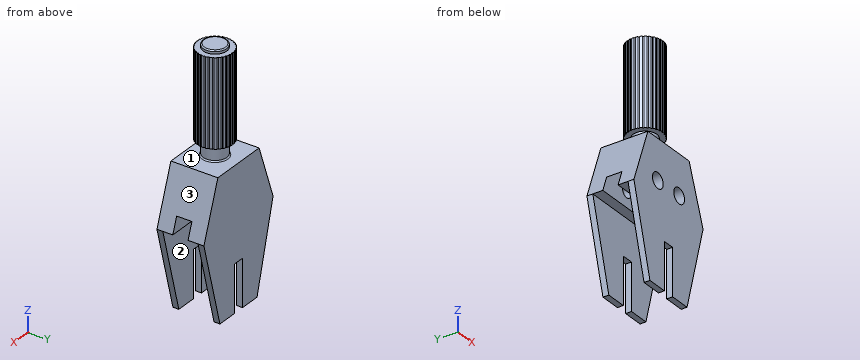
```python
from build123d import *

# Parameters (mm, degrees)
F1_DEPTH         = 200
F2_R             = 100
F3_DEPTH         = 900
F5_R             = 150
F6_DEPTH         = 740
F8_DEPTH         = 580
F9_R             = 65
F9_R_2           = 50
F10_DEPTH        = 100
F11_DEPTH        = 350
F13_DEPTH        = 65
F14_R            = 10
F15_W            = 11.6287115961
F15_H            = 9.4758689404
F16_DEPTH        = 740
F16_COPIES_COUNT = 30


# Not quite as in the source:
# - a pattern or mirror of a feature is missing from the dataset's text; its kind, count and spacing are read off the source's solid


with BuildPart() as f1:
    # F0 (on Front) → F1 (new body, symmetric)
    with BuildSketch(Plane.XZ):
        Polygon((250, 794.9763654469), (-250, 794.9763654469), (-419.1142838269, 324.4443697168), (-225, -400), (-50, -400), (-50, 0), (0, 0), (50, 0), (50, -400), (225, -400), (419.1142838269, 324.4443697168), align=None)
    extrude(amount=F1_DEPTH, both=True)

    # F2 (on face) → F3 (join)
    with BuildSketch(Plane.XY.offset(794.9763654469)):
        Circle(F2_R)
    extrude(amount=F3_DEPTH)

    # F5 (on offset) → F6 (join)
    with BuildSketch(Plane.XY.offset(924.9763654469)):
        Circle(F5_R)
    extrude(amount=F6_DEPTH)

    # F7 (on Right) → F8 (cut, symmetric)
    with BuildSketch(Plane.YZ):
        Polygon((-150, 324.4443697168), (-150, -400), (150, -400), (150, 324.4443697168), (65, 324.4443697168), (65, 454.4443697168), (-65, 454.4443697168), (-65, 324.4443697168), align=None)
    extrude(amount=F8_DEPTH, both=True, mode=Mode.SUBTRACT)

    # F9 (on face) → F10 (cut)
    with BuildSketch(Plane.XZ.offset(200)):
        with Locations((-129.1142838269, 454.4443697168)):
            Circle(F9_R)
        with Locations((-129.1142838269, 454.4443697168)):
            Circle(F9_R_2, mode=Mode.SUBTRACT)
        with Locations((129.1142838269, 454.4443697168)):
            Circle(F9_R)
        with Locations((129.1142838269, 454.4443697168)):
            Circle(F9_R_2, mode=Mode.SUBTRACT)
    extrude(amount=-F10_DEPTH, mode=Mode.SUBTRACT)

    # F11 (cut): faces of the model
    f11_faces = [f1.faces().sort_by_distance(p)[0] for p in [
        (-129.1142838269, -200, 454.4443697168),
        (129.1142838269, -200, 454.4443697168),
    ]]
    extrude(f11_faces, amount=-F11_DEPTH, mode=Mode.SUBTRACT)

    # F12 (on Front) → F13 (cut, symmetric)
    with BuildSketch(Plane.XZ):
        Polygon((272.5361245925, 584.4443697168), (-272.5361245925, 584.4443697168), (-297.6948810114, 514.4443697168), (-372.3908790489, 454.4443697168), (-419.1142838269, 324.4443697168), (419.1142838269, 324.4443697168), (372.3908790489, 454.4443697168), (297.6948810114, 514.4443697168), align=None)
    extrude(amount=F13_DEPTH, both=True, mode=Mode.SUBTRACT)

    # F14
    f14_edges = [f1.edges().sort_by_distance(p)[0] for p in [
        (-100, 0, 1694.976365),
        (-100, 0, 794.976365),
    ]]
    fillet(f14_edges, radius=F14_R)

    # F15 (on face) → F16 (cut, through all)
    with BuildSketch(Plane.XY.offset(1664.9763654469)):
        with Locations((0, 150)):
            Rectangle(F15_W, F15_H)
    f16 = extrude(amount=-F16_DEPTH, mode=Mode.SUBTRACT)

    # F16_copies: F16 ×30 about axis
    f16_copies_axis = Axis((0, 0, 0), (0, 0, 1))
    for i in range(1, F16_COPIES_COUNT):
        add(f16.rotate(f16_copies_axis, i * 360 / F16_COPIES_COUNT), mode=Mode.SUBTRACT)


solid = f1.part
```
Check sheet for the modelled part. Datum: model origin and axes. Units: mm. Face numbers are marked on the shaded views. A direction names the side the tool comes from. Round coordinates to 2 decimals unless told otherwise and drop trailing zeros. Loops run counter-clockwise (first coordinate to the right, second up) from the corner with the lowest first, then second, coordinate; pieces in that order, holes last. Notation, with made-up numbers: (-30.75, 29) -> (-5.75, 29) arc R16 ccw to (-5.75, 60) -> close; hole circle Ø3 at (80.25, 72). An arc over 180 degrees is marked (long way). Write item = value, one per line. Start each with the question number.
1) Sectioned sample at D-D, the plane z = 673. Record the cut outline in (x, y), plus the area to 3 significant figures.
2) Thickness scan on probe 1 along X at (y, z) = (-107.5, 471.5); probe 2 along Z at (x, y) = (-115.5, 76); probe 3 along Y at (x, z) = (39, 159.5). Record the ranges inside material, lowest first.
3) Set-up check for the marked faces 1, 2 and 3: record each of +Z, -Z, +X, -X, +Y, -Y from which the full face is reachable in a straight line by a thin tool's end or side.
4) Sectioned sample at A-A, the plane z = 135.5. Record the cut outline in (x, y).
5) Sectioned sample at B-B, the plane z = -74. Record the cut outline in (x, y).
6) Gauge pin test, flat ends, axial feed: pin 1 Ø8 at (y, z) = (29.5, 1230.5) entering from +X; pin 2 Ø10 at (x, y) = (107.5, 29.5) entering from -Z; pin 3 Ø10 at (y, z) = (107, 480) entering from -X. Record the tip position at first contact, or that the pin passes through.
7) Sectioned sample at C-C, the plane x = -332. Record the cut outline in (y, z).
Results are:
q1.outline = (-293.84, -200) -> (293.84, -200) -> (293.84, 200) -> (-293.84, 200) -> close
q1.area = 235,000 mm^2
q2.probe_1 = -366.26 to -191.84, -66.39 to 66.39, 191.84 to 366.26
q2.probe_2 = 324.44 to 406.33, 502.56 to 794.98, 924.98 to 1664.98
q2.probe_3 = -200 to -150, 150 to 200
q3.face_1 = none
q3.face_2 = -Z, +X, -X
q3.face_3 = +Z, +X, +Y, -Y
q4.outline = (-368.49, -200) -> (368.49, -200) -> (368.49, -150) -> (-368.49, -150) -> close; (-368.49, 150) -> (368.49, 150) -> (368.49, 200) -> (-368.49, 200) -> close
q5.outline = (-312.35, -200) -> (-50, -200) -> (-50, -150) -> (-312.35, -150) -> close; (-312.35, 150) -> (-50, 150) -> (-50, 200) -> (-312.35, 200) -> close; (50, -200) -> (312.35, -200) -> (312.35, -150) -> (50, -150) -> close; (50, 150) -> (312.35, 150) -> (312.35, 200) -> (50, 200) -> close
q6.pin_1 = 147.82
q6.pin_2 = 584.44
q6.pin_3 = -365
q7.outline = (-200, -0.67) -> (-150, -0.67) -> (-150, 324.44) -> (-65, 324.44) -> (-65, 486.89) -> (65, 486.89) -> (65, 324.44) -> (150, 324.44) -> (150, -0.67) -> (200, -0.67) -> (200, 566.83) -> (-200, 566.83) -> close
